Part model, mm, in its own coordinate system. A direction names the side the tool comes from. Give positions to 0.01 mm unless a question says otherwise; leave off trailing zeros. Order: outer loops, then holes, each group sorted by start corner. A loop starts at its lowest first (then second) coordinate and runs counter-clockwise, first axis right, second up. Notation, with made-up numbers: (53, 55) -> (68, 55) arc R21 cw to (68, 67) -> close; hole circle Ø8 at (-17, 88). An arc over 180 degrees is marked (long way). Write item = value, one per line. Start each with the question number.
(1) Which spindle directions (+Z, -Z, +X, -X, +Y, -Y) get a long thin tool onto all of the face, cutting with end or side? Do faces 1 (the cylindrical face through (12.228, -5.278, -0.542)), 2 (the cylindrical face through (14.753, -3.08, 4.872)), 3 (the flat face through (5.1, -5.5, -1.1)), 4 (the flat face through (17.73, -8.01, 5.16)). Say none if no direction does.
(2) Saw through at C-C, the plane y = -1.5. List the corners of the cut face in (x, z), then the cut area to 3 significant figures.
(3) Flat gauge pin, fed straight in: pin 1 (0.5 mm diameter, centred on x = 15, y = -3, fed in from +Z). Where does the tip first touch, or does it go through?
(4) Saw through at D-D, the plane z = 5.75. State how many separate pieces and enclosed holes the cut face has, then the cut area to 3 significant figures.
(5) Probe line 1 along Y through (x, z) = (28, 7); line 2 along Y through (x, z) = (5.5, 4); line 3 along X through (y, z) = (-3.25, 8). List the from-to ranges inside material, lowest first. Write a range as from..to.
(6) Saw through at B-B, the plane x = 24.5. List the corners of the cut face in (y, z), then the cut area to 3 significant figures.
(7) Saw through at A-A, the plane z = 7.75. List the corners of the cut face in (x, y).
from build123d import *

# Parameters (mm, degrees)
SKETCH_1_W          = 33
SKETCH_1_H          = 8.4
EXTRUDE_1_DEPTH     = 8.9
SKETCH_2_W          = 31.4
SKETCH_2_H          = 6.8
CUT_EXTRUDE_1_DEPTH = 6
CUT_EXTRUDE_2_REACH = 37.196
SKETCH_4_R          = 0.5
EXTRUDE_2_DEPTH     = 4


with BuildPart() as part:
    # 草图1 → 凸台-拉伸1 (new body)
    with BuildSketch(Plane.XY):
        with Locations((16.5, -4.2)):
            Rectangle(SKETCH_1_W, SKETCH_1_H)
    extrude(amount=EXTRUDE_1_DEPTH)

    # 草图2 → 切除-拉伸1 (cut)
    with BuildSketch(Plane.XY.offset(8.9)):
        with Locations((16.5, -4.2)):
            Rectangle(SKETCH_2_W, SKETCH_2_H)
    extrude(amount=-CUT_EXTRUDE_1_DEPTH, mode=Mode.SUBTRACT)

    # 草图3 → 切除-拉伸2 (cut, up to next)
    with BuildSketch(Plane.XZ.offset(8.4), mode=Mode.PRIVATE) as cut_extrude_2_sk1:
        Polygon((14, 8.9), (14, 6.36), (16.5, 4), (19, 6.36), (19, 8.9), align=None)
    cut_extrude_2_tool1 = extrude(cut_extrude_2_sk1.sketch, amount=-CUT_EXTRUDE_2_REACH, mode=Mode.PRIVATE) & part.part
    add(cut_extrude_2_tool1.solids().sort_by_distance((16.5, -8.4, 6.977616))[0], mode=Mode.SUBTRACT)

    # 草图4 → 凸台-拉伸2 (add, symmetric)
    with BuildSketch(Plane.XY.offset(2.9)):
        with Locations(Location((20.31, -5.47, 0), (0, 0, 180))):
            Circle(SKETCH_4_R)
        with Locations(Location((17.77, -2.93, 0), (0, 0, 180))):
            Circle(SKETCH_4_R)
        with Locations(Location((20.31, -2.93, 0), (0, 0, 180))):
            Circle(SKETCH_4_R)
        with Locations(Location((22.85, -5.47, 0), (0, 0, 180))):
            Circle(SKETCH_4_R)
        with Locations(Location((22.85, -2.93, 0), (0, 0, 180))):
            Circle(SKETCH_4_R)
        with Locations(Location((25.39, -5.47, 0), (0, 0, 180))):
            Circle(SKETCH_4_R)
        with Locations(Location((17.77, -5.47, 0), (0, 0, 180))):
            Circle(SKETCH_4_R)
        with Locations(Location((25.39, -2.93, 0), (0, 0, 180))):
            Circle(SKETCH_4_R)
        with Locations(Location((27.93, -5.47, 0), (0, 0, 180))):
            Circle(SKETCH_4_R)
        with Locations(Location((27.93, -2.93, 0), (0, 0, 180))):
            Circle(SKETCH_4_R)
        with Locations(Location((5.07, -2.93, 0), (0, 0, 180))):
            Circle(SKETCH_4_R)
        with Locations(Location((5.07, -5.47, 0), (0, 0, 180))):
            Circle(SKETCH_4_R)
        with Locations(Location((7.61, -5.47, 0), (0, 0, 180))):
            Circle(SKETCH_4_R)
        with Locations(Location((7.61, -2.93, 0), (0, 0, 180))):
            Circle(SKETCH_4_R)
        with Locations(Location((10.15, -2.93, 0), (0, 0, 180))):
            Circle(SKETCH_4_R)
        with Locations(Location((10.15, -5.47, 0), (0, 0, 180))):
            Circle(SKETCH_4_R)
        with Locations(Location((12.69, -5.47, 0), (0, 0, 180))):
            Circle(SKETCH_4_R)
        with Locations(Location((12.69, -2.93, 0), (0, 0, 180))):
            Circle(SKETCH_4_R)
        with Locations(Location((15.23, -2.93, 0), (0, 0, 180))):
            Circle(SKETCH_4_R)
        with Locations(Location((15.23, -5.47, 0), (0, 0, 180))):
            Circle(SKETCH_4_R)
    extrude(amount=EXTRUDE_2_DEPTH, both=True)


solid = part.part
Results list:
q1.face_1 = -Z
q1.face_2 = +Z
q1.face_3 = -Z, +X, -X, +Y, -Y
q1.face_4 = +Z, -Y
q2.outline = (0, 0) -> (33, 0) -> (33, 8.9) -> (32.2, 8.9) -> (32.2, 2.9) -> (0.8, 2.9) -> (0.8, 8.9) -> (0, 8.9) -> close
q2.area = 105 mm^2
q3.pin_1 = 6.9
q4.separate_pieces = 21
q4.enclosed_holes = 0
q4.area = 76.4 mm^2
q5.line_1 = -8.4..-7.6, -0.8..0
q5.line_2 = -8.4..-7.6, -5.73..-5.21, -3.19..-2.67, -0.8..0
q5.line_3 = 0..0.8, 32.2..33
q6.outline = (-8.4, 0) -> (0, 0) -> (0, 8.9) -> (-0.8, 8.9) -> (-0.8, 2.9) -> (-7.6, 2.9) -> (-7.6, 8.9) -> (-8.4, 8.9) -> close
q6.area = 34.0 mm^2
q7.outline = (0, -8.4) -> (14, -8.4) -> (14, -7.6) -> (0.8, -7.6) -> (0.8, -0.8) -> (32.2, -0.8) -> (32.2, -7.6) -> (19, -7.6) -> (19, -8.4) -> (33, -8.4) -> (33, 0) -> (0, 0) -> close
